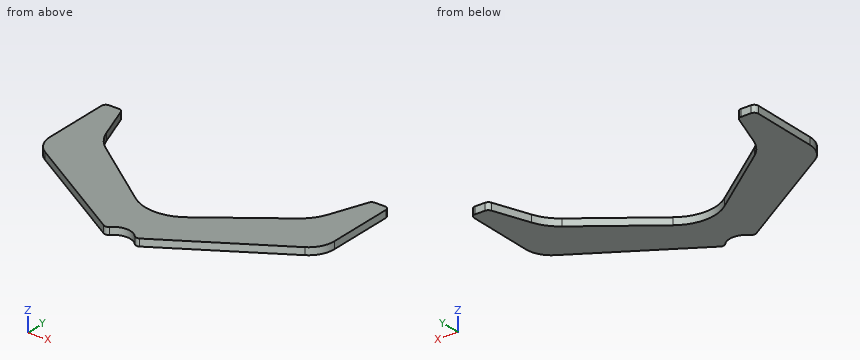
```python
from build123d import *

# Parameters (mm, degrees)
BASE_EXTRUDE_DEPTH = 5


with BuildPart() as part:
    # Sketch1 → Base-Extrude (new body)
    with BuildSketch(Plane.XY):
        with BuildLine():
            Line((-99, 117), (-99, 70.747762378))
            ThreePointArc((-99, 70.747762378), (-96.704928127, 61.952580031), (-90.404974165, 55.40023942))
            Line((-90.404974165, 55.40023942), (-12.531200021, 7.679129249))
            ThreePointArc((-12.531200021, 7.679129249), (-10.560110304, 7.264321725), (-8.770963462, 8.189639794))
            ThreePointArc((-8.770963462, 8.189639794), (0, 12), (8.770963462, 8.189639794))
            ThreePointArc((8.770963462, 8.189639794), (10.560110304, 7.264321725), (12.531200021, 7.679129249))
            Line((12.531200021, 7.679129249), (90.404974165, 55.40023942))
            ThreePointArc((90.404974165, 55.40023942), (96.704928127, 61.952580031), (99, 70.747762378))
            Line((99, 70.747762378), (99, 117))
            ThreePointArc((99, 117), (98.121320344, 119.121320344), (96, 120))
            Line((96, 120), (89.100622615, 120))
            ThreePointArc((89.100622615, 120), (87.379893306, 119.457456133), (86.281544752, 118.02606043))
            Line((86.281544752, 118.02606043), (77.324366423, 93.416415229))
            ThreePointArc((77.324366423, 93.416415229), (73.17120218, 85.727281512), (66.978271402, 79.56131371))
            Line((66.978271402, 79.56131371), (17.844683603, 43.204371262))
            ThreePointArc((17.844683603, 43.204371262), (0, 37.320077081), (-17.844683603, 43.204371262))
            Line((-17.844683603, 43.204371262), (-66.978271402, 79.56131371))
            ThreePointArc((-66.978271402, 79.56131371), (-73.17120218, 85.727281512), (-77.324366423, 93.416415229))
            Line((-77.324366423, 93.416415229), (-86.281544752, 118.02606043))
            ThreePointArc((-86.281544752, 118.02606043), (-87.379893306, 119.457456133), (-89.100622615, 120))
            Line((-89.100622615, 120), (-96, 120))
            ThreePointArc((-96, 120), (-98.121320344, 119.121320344), (-99, 117))
        make_face()
    extrude(amount=BASE_EXTRUDE_DEPTH)


solid = part.part
```
Input: part model. Units: mm. Frame: model coordinates. Coordinates: 2 decimals unless noted, no trailing zeros. Order: outer loops, then holes, each group sorted by start corner. A loop starts at its lowest first (then second) coordinate and runs counter-clockwise, first axis right, second up. Notation, with made-up numbers: (80, 47.25) - (133, 47.25) arc R15 cw to (133, 69.25) - close; hole circle Ø9 at (63.25, 59.5). An arc over 180 degrees is marked (long way). Put each result on its own line as item: value.
1. Cut plane A-A on y = 103.5. Return the cut outline in (x, z), then the cut area to 3 significant figures.
Report:
outline: (-99, 0) - (-80.99, 0) - (-80.99, 5) - (-99, 5) - close; (80.99, 0) - (99, 0) - (99, 5) - (80.99, 5) - close
area: 180 mm2
2. Cut plane C-C on y = 68. Return the cut outline in (x, z), then the cut area to 3 significant figures.
Report:
outline: (-98.79, 0) - (-51.35, 0) - (-51.35, 5) - (-98.79, 5) - close; (51.35, 0) - (98.79, 0) - (98.79, 5) - (51.35, 5) - close
area: 474 mm2
3. Contact query for flat-ended pins moving along their axis: pin 1 Ø3 at (x, z) = (-67, 3) entering from +Y; pin 2 Ø3 at (x, z) = (44, 3.5) entering from +Y. Output: stop coordinate, or through.
Report:
pin 1: stops at y = 80.77
pin 2: stops at y = 63.67
4. Line query: line 1 along Y through (x, z) = (0, 2); line 2 along X through (y, z) = (80.5, 0.55); line 3 along X through (y, z) = (70.5, 0.8). Output: solid intervals per line, ascending.
Report:
line 1: y = 12 to 37.32
line 2: x = -99 to -68.18, 68.18 to 99
line 3: x = -99 to -54.73, 54.73 to 99
5. Cut plane B-B on z = 3.85. Return the cut outline in (x, y).
Report:
outline: (-99, 70.75) arc R18 ccw to (-90.4, 55.4) - (-12.53, 7.68) arc R3 ccw to (-8.77, 8.19) arc R12 cw to (8.77, 8.19) arc R3 ccw to (12.53, 7.68) - (90.4, 55.4) arc R18 ccw to (99, 70.75) - (99, 117) arc R3 ccw to (96, 120) - (89.1, 120) arc R3 ccw to (86.28, 118.03) - (77.32, 93.42) arc R30 cw to (66.98, 79.56) - (17.84, 43.2) arc R30 cw to (-17.84, 43.2) - (-66.98, 79.56) arc R30 cw to (-77.32, 93.42) - (-86.28, 118.03) arc R3 ccw to (-89.1, 120) - (-96, 120) arc R3 ccw to (-99, 117) - close
6. Cut plane D-D on x = 26. Return the cut outline in (y, z).
Report:
outline: (15.93, 0) - (49.24, 0) - (49.24, 5) - (15.93, 5) - close
